```python
from build123d import *

# Parameters (mm, degrees)
F1_DEPTH = 25.4
F3_DEPTH = 25.4
F5_DEPTH = 25.4
F7_DEPTH = 25.4
F9_DEPTH = 25.4


# Not quite as in the source:
# - a feature names something its author has since deleted; it is built from what else it names


with BuildPart() as f1:
    # F0 (on Front) → F1 (new body)
    with BuildSketch(Plane.XZ):
        Polygon((-5.5358944303, 38.1), (-30.9358944303, 38.1), (-30.9358944303, 0), (38.9141055698, 0), (38.9141055697, 12.7), (-5.5358944303, 12.7), align=None)
    extrude(amount=F1_DEPTH)

    # F2 (on face) → F3 (cut)
    with BuildSketch(Plane.XY.offset(38.1)):
        with BuildLine():
            ThreePointArc((-11.8858944302, -12.7), (-13.7457663697, -8.2098719395), (-18.2358944302, -6.35))
            Line((-18.2358944303, -6.35), (-18.2358944303, -12.7))
            Line((-18.2358944302, -12.7), (-11.8858944302, -12.7))
        make_face()
        with BuildLine():
            Line((-11.8858944302, -12.7), (-18.2358944302, -12.7))
            Line((-18.2358944303, -12.7), (-18.2358944303, -19.05))
            ThreePointArc((-18.2358944302, -19.05), (-13.7457663697, -17.1901280605), (-11.8858944302, -12.7))
        make_face()
        with BuildLine():
            Line((-18.2358944302, -12.7), (-24.5858944303, -12.7))
            ThreePointArc((-24.5858944303, -12.7), (-22.7260224908, -17.1901280605), (-18.2358944302, -19.05))
            Line((-18.2358944303, -19.05), (-18.2358944303, -12.7))
        make_face()
        with BuildLine():
            Line((-18.2358944303, -12.7), (-18.2358944303, -6.35))
            ThreePointArc((-18.2358944302, -6.35), (-22.7260224908, -8.2098719395), (-24.5858944303, -12.7))
            Line((-24.5858944303, -12.7), (-18.2358944302, -12.7))
        make_face()
        with BuildLine():
            Line((-5.5358944303, 0), (-18.2358944303, 0))
            ThreePointArc((-18.2358944303, 0), (-9.2556383092, -3.7197438789), (-5.5358944303, -12.7))
            Line((-5.5358944303, -12.7), (-5.5358944303, 0))
        make_face()
        with BuildLine():
            Line((-5.5358944303, -25.4), (-5.5358944303, -12.7))
            ThreePointArc((-5.5358944303, -12.7), (-9.2556383092, -21.6802561211), (-18.2358944303, -25.4))
            Line((-18.2358944303, -25.4), (-5.5358944303, -25.4))
        make_face()
    extrude(amount=-F3_DEPTH, mode=Mode.SUBTRACT)

    # F4 (on face) → F5 (cut)
    with BuildSketch(Plane.XY.offset(12.7)):
        with BuildLine():
            Line((29.3793692031, -9.1760675128), (10.3391055697, -9.0105000585))
            Line((10.3391055697, -9.0105000585), (10.3391055697, -16.195377335))
            Line((10.3391055697, -16.195377335), (29.3492708089, -16.195377335))
            ThreePointArc((29.3492708089, -16.195377335), (26.7811699001, -12.6746460258), (29.3793692031, -9.1760675128))
        make_face()
        with BuildLine():
            Line((10.3391055697, -16.195377335), (10.3391055697, -9.0105000585))
            Line((10.3391055697, -9.0105000585), (3.7719008779, -8.9533939498))
            ThreePointArc((3.7719008779, -8.9533939498), (5.7024746114, -10.3218470376), (6.442491519, -12.5695466995))
            ThreePointArc((6.442491519, -12.5695466995), (5.6925301995, -14.8306497777), (3.7399555387, -16.195377335))
            Line((3.7399555387, -16.195377335), (10.3391055697, -16.195377335))
        make_face()
        with BuildLine():
            ThreePointArc((34.132825273, -12.6904076897), (32.6422382322, -9.7346534929), (29.3793692031, -9.1760675128))
            Line((29.3793692031, -9.1760675128), (30.4569806904, -9.1854380444))
            Line((30.4569806904, -9.1854380444), (30.4569806904, -16.195377335))
            Line((30.4569806904, -16.195377335), (29.3492708089, -16.195377335))
            ThreePointArc((29.3492708089, -16.195377335), (32.6295441565, -15.6555048856), (34.132825273, -12.6904076897))
        make_face()
        with BuildLine():
            Line((30.4569806904, -9.1854380444), (29.3793692031, -9.1760675128))
            ThreePointArc((29.3793692031, -9.1760675128), (26.7811699001, -12.6746460258), (29.3492708089, -16.195377335))
            Line((29.3492708089, -16.195377335), (30.4569806904, -16.195377335))
            Line((30.4569806904, -16.195377335), (30.4569806904, -9.1854380444))
        make_face()
        with BuildLine():
            ThreePointArc((6.442491519, -12.5695466995), (5.7024746114, -10.3218470376), (3.7719008779, -8.9533939498))
            Line((3.7719008779, -8.9533939498), (2.6589436457, -8.9437160641))
            Line((2.6589436457, -8.9437160641), (2.6589436457, -16.195377335))
            Line((2.6589436457, -16.195377335), (3.7399555387, -16.195377335))
            ThreePointArc((3.7399555387, -16.195377335), (5.6925301995, -14.8306497777), (6.442491519, -12.5695466995))
        make_face()
        with BuildLine():
            Line((2.6589436457, -8.9437160641), (3.7719008779, -8.9533939498))
            ThreePointArc((3.7719008779, -8.9533939498), (-1.1245674179, -12.5528571357), (3.7399555387, -16.195377335))
            Line((3.7399555387, -16.195377335), (2.6589436457, -16.195377335))
            Line((2.6589436457, -16.195377335), (2.6589436457, -8.9437160641))
        make_face()
    extrude(amount=-F5_DEPTH, mode=Mode.SUBTRACT)

    # F6 (on face) → F7 (cut)
    with BuildSketch(Plane.XY.offset(12.7)):
        with BuildLine():
            Line((38.9141055697, -12.7), (38.9141055697, 0))
            Line((38.9141055697, 0), (26.2141055698, 0))
            ThreePointArc((26.2141055698, 0), (35.1943616908, -3.7197438789), (38.9141055697, -12.7))
        make_face()
    extrude(amount=-F7_DEPTH, mode=Mode.SUBTRACT)

    # F8 (on face) → F9 (cut)
    with BuildSketch(Plane.XY.offset(12.7)):
        with BuildLine():
            Line((38.9141055697, -25.4), (38.9141055697, -12.7))
            ThreePointArc((38.9141055697, -12.7), (35.1943616908, -21.6802561211), (26.2141055698, -25.4))
            Line((26.2141055698, -25.4), (38.9141055697, -25.4))
        make_face()
    extrude(amount=-F9_DEPTH, mode=Mode.SUBTRACT)


solid = f1.part
```
The listing builds one solid part. Answer for the finished solid, in the listing's coordinates (mm). A direction names the side the tool comes from. Coordinates: 2 decimals unless noted, no trailing zeros. Write each loop counter-clockwise with the first axis right and the second up, starting at its lowest first coordinate (ties: lowest second). Pieces come first, ordered by that corner, then holes. Notation, with made-up numbers: (43.5, 70.25) - (48.5, 70.25) arc R20 cw to (48.5, 74.25) - close; hole circle Ø9 at (46, 83). An arc over 180 degrees is marked (long way). Return JSON: item names as keys, results as strings. Group by question number.
Q1. The part is cut by section C-C on x = 12. Write down the section's boundary in (y, z).
Q2. Flat-ended cylindrical pins translate along their axes: pin 1 Ø4 at (x, y) = (-19.5, -13.5) entering from +Z; pin 2 Ø8 at (y, z) = (-12, 30.5) entering from +X; pin 3 Ø3 at (x, z) = (-12.5, 17.5) entering from -Y; pin 4 Ø4 at (x, y) = (-3.5, -19) entering from -Z. Find the tip coordinate at first contact, or state that the pin passes through.
Q3. The part is cut by section D-D on z = 7. Write down the section's boundary in (x, y), and give its area (3 significant figures).
Q4. The part is cut by section B-B on y = -11.25. Write down the section's boundary in (x, z).
Q5. Find the intervals of material crossed by line 1 along Z through (x, y) = (-1, -9.75); line 2 along X through (y, z) = (-9.75, 19.5); line 3 along X through (y, z) = (-13.25, 18.5), in increasing order. Write a range as [from, to].
Q6. For a pull along Y with two mould halves and no side action, classify faces 1 (the flat face through (16, -7, 12.7)), 2 (the flat face through (-9, 0, 11)), 3 (the flat face through (-18, -13, 12.7)) as +Y half, -Y half, draft (parallel to the pull), parting line (faces both ways), or undercut.
Q7. The part is cut by section A-A on z = 16.5. Write down the section's boundary in (x, y).
Q8. Which of the six approach directions +Z, -Z, +X, -X, +Y, -Y give full straight-line access (tool end or side, diameter ignored) to faces 4 (the flat face through (16, -16.195, 6)), 5 (the flat face through (-9, -25.4, 11))?
Evaluation:
{
 "1": {"outline": "(-25.4, 0) - (-16.2, 0) - (-16.2, 12.7) - (-25.4, 12.7) - close; (-9.02, 0) - (0, 0) - (0, 12.7) - (-9.02, 12.7) - close"},
 "2": {"pin 1": "stops at z = 12.7", "pin 2": "stops at x = -5.54", "pin 3": "stops at y = -24.67", "pin 4": "stops at z = 0"},
 "3": {"outline": "(-30.94, -25.4) - (26.21, -25.4) arc R12.7 ccw to (26.21, 0) - (-30.94, 0) - close; hole (3.74, -16.2) - (29.35, -16.2) arc R3.68 ccw (long way) to (29.38, -9.18) - (3.77, -8.95) arc R3.78 ccw (long way) to start", "area": "1,460 mm2"},
 "4": {"outline": "(-30.94, 0) - (-0.89, 0) - (-0.89, 12.7) - (-5.62, 12.7) - (-5.62, 38.1) - (-12.05, 38.1) - (-12.05, 12.7) - (-24.42, 12.7) - (-24.42, 38.1) - (-30.94, 38.1) - close; (33.84, 0) - (38.83, 0) - (38.83, 12.7) - (33.84, 12.7) - close"},
 "5": {"line 1": "z = [0, 12.7]", "line 2": "x = [-30.94, -23.86], [-12.61, -5.88]", "line 3": "x = [-30.94, -24.56], [-11.91, -5.55]"},
 "6": {"face 1": "draft", "face 2": "+Y half", "face 3": "undercut"},
 "7": {"outline": "(-30.94, -25.4) - (-18.24, -25.4) arc R12.7 ccw to (-18.24, 0) - (-30.94, 0) - close; hole circle Ø12.7 at (-18.24, -12.7)"},
 "8": {"face 4": "+Z, -Z", "face 5": "+Z, -Z, +X, -X, -Y"}
}
